```python
from build123d import *

# Parameters (mm, degrees)
CYLINDER003_R     = 2
CYLINDER003_DEPTH = 10
ARRAY001_COUNT    = 8
CYLINDER002_R     = 10
CYLINDER002_DEPTH = 30
CYLINDER_R        = 30
CYLINDER_DEPTH    = 5
CYLINDER001_R     = 15
CYLINDER001_DEPTH = 12


with BuildPart() as array001:
    # Cylinder003 → Cylinder003 (new body)
    with BuildSketch(Plane(origin=(22, 0, -2), x_dir=(1, 0, 0), z_dir=(0, 0, 1))):
        Circle(CYLINDER003_R)
    extrude(amount=CYLINDER003_DEPTH)

    # Array001: Array001 ×8 about axis
    array001_axis = Axis((0, 0, 1), (0, 0, 1))


with BuildPart() as array001_1:
    add(array001.part)
    for i in range(1, ARRAY001_COUNT):
        add(array001.part.rotate(array001_axis, i * 360 / ARRAY001_COUNT))


with BuildPart() as int:
    # Cylinder002 → Cylinder002 (new body)
    with BuildSketch(Plane.XY.offset(-2)):
        Circle(CYLINDER002_R)
    extrude(amount=CYLINDER002_DEPTH)


with BuildPart() as basis:
    # Cylinder → Cylinder (new body)
    with BuildSketch(Plane.XY):
        Circle(CYLINDER_R)
    extrude(amount=CYLINDER_DEPTH)


with BuildPart() as flange:
    # Cylinder001 → Cylinder001 (new body)
    with BuildSketch(Plane.XY):
        Circle(CYLINDER001_R)
    extrude(amount=CYLINDER001_DEPTH)

    # Fusion: union basis
    add(basis.part)

    # Cut: cut int
    add(int.part, mode=Mode.SUBTRACT)

    # Cut001: cut Array001
    add(array001_1.part, mode=Mode.SUBTRACT)


solid = flange.part
```
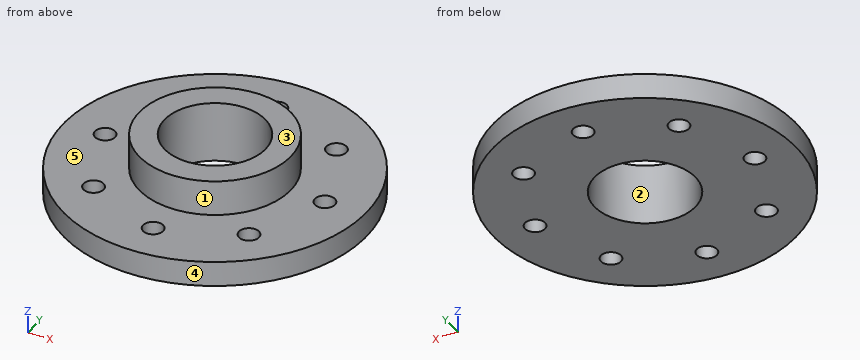
Verification items for the finished model (mm, model axes). Face numbers are marked on the shaded views. A direction names the side the tool comes from. Round coordinates to 2 decimals unless told otherwise and drop trailing zeros. Order: outer loops, then holes, each group sorted by start corner. A loop starts at its lowest first (then second) coordinate and runs counter-clockwise, first axis right, second up. Notation, with made-up numbers: (-28.75, 27) - (-20.75, 27) arc R11 ccw to (-20.75, 33) - close; hole circle Ø11 at (-28.5, 31). An arc over 180 degrees is marked (long way). Use CSV: the item, a comma, the result in double quotes. Start each with the question number.
1) Thickness scan on L1, parallel to Y at x = -15.5, z = 2; L2, parallel to Y at x = 0.5, z = 5.25; L3, parallel to Z at x = -24, y = 10. Record the ranges inside material, lowest first.
2) Section check C-C, the plane y = 21. Record the cut outline in (x, z), plus the area to 3 significant figures.
3) Go/stop test with flat-tipped pins: P1, Ø1.5, axis at y = 19.5, z = 5.5, coming from the -X side; P2, Ø5, axis at x = 0, y = 22, coming from the +Z side; P3, Ø1, axis at y = 12, z = 10.5, coming from the +X side; P4, Ø2, axis at x = 8, y = 5, coming from the -Z side. Record where each tip stops, or that it passes through.
4) Access from +Z, -Z, +X, -X, +Y, -Y to the whole of each face (thin tool, end or side, straight path). Record for the marked faces 4 and 5.
5) Mould release check, pull along Y, two halves, no side actions. Record for the marked faces 1, 2 and 3: +Y half, -Y half, draft (parallel to the pull), parting line (faces both ways), or undercut.
6) Section check D-D, the plane x = -22. Record the cut outline in (y, z).
7) Section check A-A, the plane y = 0. Record the cut outline in (x, z).
Answers:
1,L1,"y = -25.69 to -17.56, -13.56 to 13.56, 17.56 to 25.69"
1,L2,"y = -14.99 to -9.99, 9.99 to 14.99"
1,L3,"z = 0 to 5"
2,outline,"(-21.42, 0) - (-1.73, 0) - (-1.73, 5) - (-21.42, 5) - close; (1.73, 0) - (21.42, 0) - (21.42, 5) - (1.73, 5) - close"
2,area,"197 mm²"
3,P1,"stops at x = -23.26"
3,P2,"stops at z = 5"
3,P3,"stops at x = 9.63"
3,P4,"stops at z = 0"
4,face 4,"+Z, -Z"
4,face 5,"+Z"
5,face 1,"parting line"
5,face 2,"undercut"
5,face 3,"draft"
6,outline,"(-20.4, 0) - (-2, 0) - (-2, 5) - (-20.4, 5) - close; (2, 0) - (20.4, 0) - (20.4, 5) - (2, 5) - close"
7,outline,"(-30, 0) - (-24, 0) - (-24, 5) - (-30, 5) - close; (-20, 0) - (-10, 0) - (-10, 12) - (-15, 12) - (-15, 5) - (-20, 5) - close; (10, 0) - (20, 0) - (20, 5) - (15, 5) - (15, 12) - (10, 12) - close; (24, 0) - (30, 0) - (30, 5) - (24, 5) - close"
